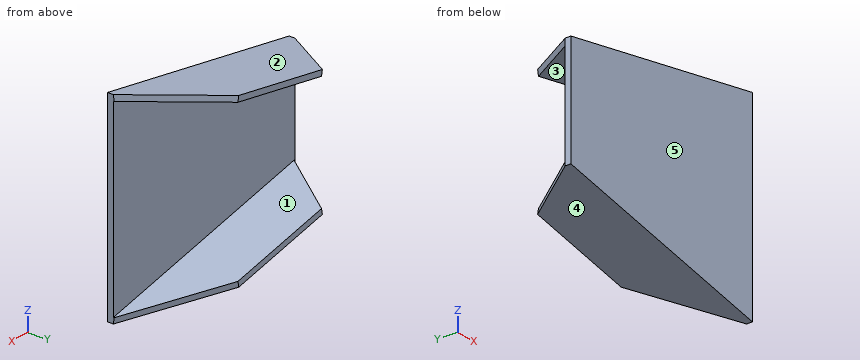
```python
from build123d import *

# Parameters (mm, degrees)
BOSS_EXTRUDE1_DEPTH = 2
BOSS_EXTRUDE2_DEPTH = 20
CUT_EXTRUDE6_DEPTH  = 5
CUT_EXTRUDE7_DEPTH  = 5
CUT_EXTRUDE8_DEPTH  = 5
CUT_EXTRUDE9_DEPTH  = 5


with BuildPart() as part:
    # Sketch1 → Boss-Extrude1 (new body)
    with BuildSketch(Plane(origin=(0, 0, 0), x_dir=(1, 0, 0), z_dir=(0, 1, 0))):
        Polygon((0, 0), (0, -39), (78.484074818, -54.5), (78.484074818, 15.5), align=None)
    extrude(amount=BOSS_EXTRUDE1_DEPTH)

    # Sketch2 → Boss-Extrude2 (add)
    with BuildSketch(Plane(origin=(0, 2, 0), x_dir=(1, 0, 0), z_dir=(0, 1, 0))):
        Polygon((0, -39), (78.484074818, -54.5), (78.484074818, -52.5), (0, -37), align=None)
        Polygon((78.484074818, 15.5), (78.484074818, 13.5), (0, -2), (0, 0), align=None)
    extrude(amount=BOSS_EXTRUDE2_DEPTH)

    # Sketch3 → Cut-Extrude6 (cut)
    with BuildSketch(Plane(origin=(-7.413066129, 0, 37.535976563), x_dir=(0.98105093522202, 0, 0.19375000000000017), z_dir=(-0.19375000000000017, 0, 0.98105093522202))):
        Polygon((21.046420337, 22), (2.156848068, 22), (2.156848068, 2), (7.55625, 2), align=None)
    extrude(amount=-CUT_EXTRUDE6_DEPTH, mode=Mode.SUBTRACT)

    # Sketch4 → Cut-Extrude7 (cut)
    with BuildSketch(Plane(origin=(0, 0, 0), x_dir=(-0.98105093522202, 0, 0.1937499999999999), z_dir=(-0.19374999999999987, 0, -0.9810509352220199))):
        Polygon((-13.489984999, 22), (7.971845258, 22), (7.971845258, 2.000274775), (0, 2.000274775), align=None)
    extrude(amount=-CUT_EXTRUDE7_DEPTH, mode=Mode.SUBTRACT)

    # Sketch6 → Cut-Extrude8 (cut)
    with BuildSketch(Plane(origin=(-7.413066129, 0, 37.535976563), x_dir=(0.98105093522202, 0, 0.19375000000000017), z_dir=(-0.19375000000000017, 0, 0.98105093522202))):
        Polygon((57.90503063, 22), (98.623999419, 22), (98.623999419, 2), (87.55625, 2), align=None)
    extrude(amount=-CUT_EXTRUDE8_DEPTH, mode=Mode.SUBTRACT)

    # Sketch7 → Cut-Extrude9 (cut)
    with BuildSketch(Plane(origin=(0, 0, 0), x_dir=(-0.98105093522202, 0, 0.1937499999999999), z_dir=(-0.19374999999999987, 0, -0.9810509352220199))):
        Polygon((-50.34878063, 22), (-88.981830345, 22), (-88.981830345, 2), (-80, 2), align=None)
    extrude(amount=-CUT_EXTRUDE9_DEPTH, mode=Mode.SUBTRACT)


solid = part.part
```
Geometry check sheet. Reference: the model listing, model coordinates, mm. Face numbers are marked on the shaded views. A direction names the side the tool comes from. Round coordinates to 2 decimals unless told otherwise and drop trailing zeros. Loops run counter-clockwise (first coordinate to the right, second up) from the corner with the lowest first, then second, coordinate; pieces in that order, holes last. Notation, with made-up numbers: (4.5, 47.25) -> (14.5, 47.25) arc R24 ccw to (14.5, 66.25) -> close; hole circle Ø3 at (-6, 72). An arc over 180 degrees is marked (long way). Use a Markdown table: item, result.
(1) Scan lines: probe 1 along Z at (x, y) = (35.5, 6.5); probe 2 along Z at (x, y) = (36, 18.25); probe 3 along Y at (x, z) = (47.5, 25.5). Record each from-to range of solid material in increasing order.
Calculated:
| item | result |
|---|---|
| probe 1 | -7.01 to -5.01, 44.01 to 46.01 |
| probe 2 | -7.11 to -5.11, 44.11 to 46.11 |
| probe 3 | 0 to 2 |
(2) Sectioned sample at B-B (x = 20). Enter the section's corners in (y, z).
Calculated:
| item | result |
|---|---|
| outline | (0, -3.95) -> (22, -3.95) -> (22, -1.95) -> (2, -1.95) -> (2, 40.95) -> (22, 40.95) -> (22, 42.95) -> (0, 42.95) -> close |
(3) Sectioned sample at C-C (z = 1). Enter the section's corners in (x, y), then the cut area to 3 significant figures.
Calculated:
| item | result |
|---|---|
| outline | (0, 0) -> (78.48, 0) -> (78.48, 2) -> (5.06, 2) -> (5.06, 9.08) -> (0.2, 2) -> (0, 2) -> close |
| area | 174 mm² |
(4) Set-up check for the marked faces 1 and 2: record each of +Z, -Z, +X, -X, +Y, -Y from which the full face is reachable in a straight line by a thin tool's end or side.
Calculated:
| item | result |
|---|---|
| face 1 | +X, +Y |
| face 2 | +Z, -X, +Y, -Y |
(5) Sectioned sample at D-D (y = 18.5). Enter the section's corners in (x, z), then the cut area to 3 significant figures.
Calculated:
| item | result |
|---|---|
| outline | (10.92, -2.16) -> (54.49, -10.76) -> (54.87, -8.84) -> (11.3, -0.23) -> close; (10.92, 41.16) -> (11.3, 39.23) -> (54.87, 47.84) -> (54.49, 49.76) -> close |
| area | 174 mm² |
(6) Mould release check, pull along Z, two halves, no side actions. Record for the marked faces 3, 4 and 5: released by +Z, released by -Z, zero draft, split by the parting line, or undercut.
Calculated:
| item | result |
|---|---|
| face 3 | undercut |
| face 4 | released by -Z |
| face 5 | zero draft |
(7) Go/stop test with flat-tipped pins: P1, Ø1, axis at x = 21, y = 16, coming from the -Z side; P2, Ø4, axis at y = 17, z = -3.5, coming from the -X side; P3, Ø5, axis at x = 11.5, z = 18, coming from the +Y side. Record where each tip stops, or that it passes through.
Calculated:
| item | result |
|---|---|
| P1 | z = -4.25 |
| P2 | x = 9.21 |
| P3 | y = 2 |
(8) Sectioned sample at A-A (y = 7.5). Enter the section's corners in (x, z), then the cut area to 3 significant figures.
Calculated:
| item | result |
|---|---|
| outline | (3.64, -0.72) -> (70.48, -13.92) -> (70.86, -12) -> (4.02, 1.21) -> close; (3.64, 39.72) -> (4.02, 37.79) -> (70.86, 51) -> (70.48, 52.92) -> close |
| area | 267 mm² |
